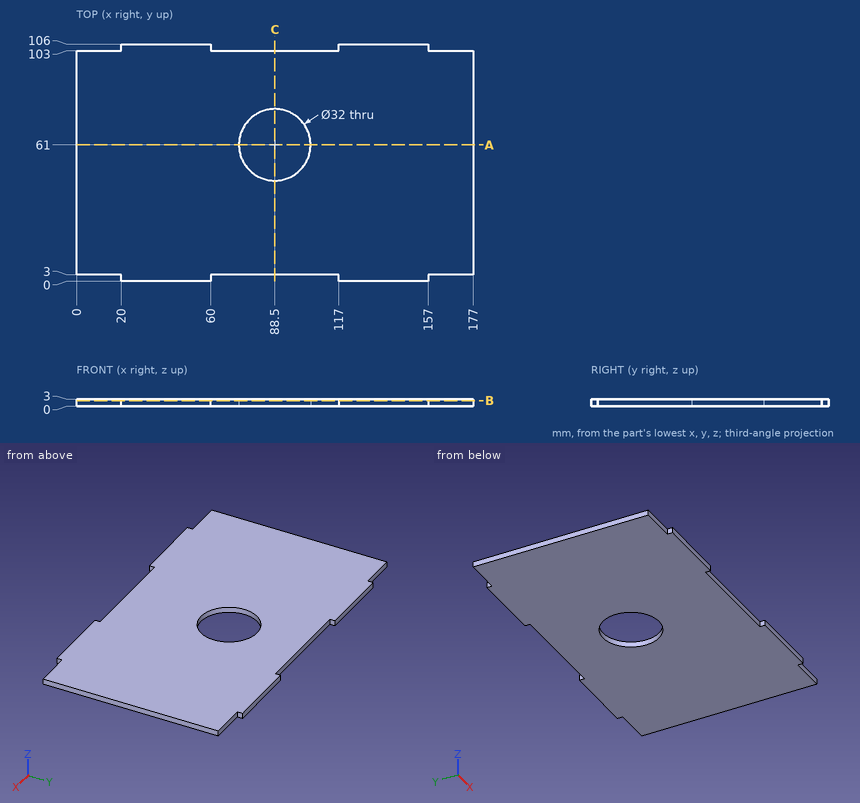
Part print with two shaded views. Sizes in mm from the minimum x, y, z corner. Round coordinates to 2 decimals unless told otherwise and drop trailing zeros. Write each loop counter-clockwise with the first axis right and the second up, starting at its lowest first coordinate (ties: lowest second). Pieces come first, ordered by that corner, then holes. Notation, with made-up numbers: (28, 13) - (77, 13) arc R21 ccw to (77, 43) - close; hole circle Ø3 at (40.25, 39.25). An arc over 180 degrees is marked (long way). Answer as CSV lines item,"result".
Q1. Drop flat-ended pins along their axis: pin 1 (1.5 mm diameter, centred on x = 168, z = 1, fed in from +Y); pin 2 (0.9 mm diameter, centred on y = 1, z = 1.5, fed in from +X); pin 3 (1.5 mm diameter, centred on y = 2, z = 2, fed in from -X). Give the stop position or say it passes through.
Report:
pin 1,"stops at y = 103"
pin 2,"stops at x = 157"
pin 3,"stops at x = 20"
Q2. Cut at A-A (y = 61). Write the cut outline in (x, z).
Report:
outline,"(0, 0) - (72.5, 0) - (72.5, 3) - (0, 3) - close; (104.5, 0) - (177, 0) - (177, 3) - (104.5, 3) - close"
Q3. Drill centre lines: probe 1 along Y at (x, z) = (88.5, 2.15); probe 2 along X at (y, z) = (47, 2.85); probe 3 along Y at (x, z) = (69, 2.8). Where is each one in solid material? Low to high. Write a range as [from, to].
Report:
probe 1,"y = [3, 45], [77, 103]"
probe 2,"x = [0, 80.75], [96.25, 177]"
probe 3,"y = [3, 103]"
Q4. Cut at C-C (x = 88.5). Write the cut outline in (y, z), and give its area (3 significant figures).
Report:
outline,"(3, 0) - (45, 0) - (45, 3) - (3, 3) - close; (77, 0) - (103, 0) - (103, 3) - (77, 3) - close"
area,"204 mm^2"
Q5. Cut at B-B (z = 2.5). Write the cut outline in (x, y).
Report:
outline,"(0, 3) - (20, 3) - (20, 0) - (60, 0) - (60, 3) - (117, 3) - (117, 0) - (157, 0) - (157, 3) - (177, 3) - (177, 103) - (157, 103) - (157, 106) - (117, 106) - (117, 103) - (60, 103) - (60, 106) - (20, 106) - (20, 103) - (0, 103) - close; hole circle Ø32 at (88.5, 61)"
